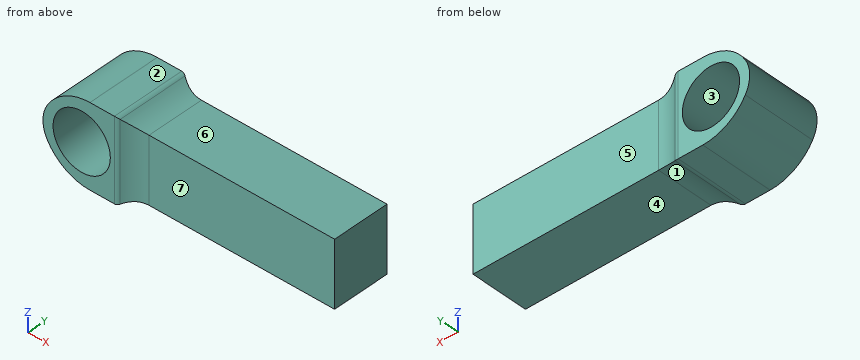
```python
from build123d import *

# Parameters (mm, degrees)
F0_W        = 10
F0_H        = 9
F1_DEPTH    = 5
F3_D        = 7
F4_T1_DEPTH = 39
F5_R        = 1
F6_W        = 7
F6_H        = 8
F7_DEPTH    = 25
F8_R        = 5
F9_R        = 4


# Not quite as in the source:
# - a fillet or chamfer that OpenCascade refuses, or shapes differently, is made with other operations: its cross-section is extruded or revolved along the edge and cut away or added


with BuildPart() as f1:
    # F0 (on Top) → F1 (new body, symmetric)
    with BuildSketch(Plane.XY):
        Rectangle(F0_W, F0_H)
    extrude(amount=F1_DEPTH, both=True)

    # F3 (through all)
    with Locations(Plane(origin=(0, 4.5, 0), x_dir=(-1, 0, 0), z_dir=(0, 1, 0))):
        with Locations((0, 0)):
            Hole(F3_D / 2)

    # F4: fillet of radius 6 on 2 edges, made by hand

    # F4_s2 → F4_t1 (cut)
    with BuildSketch(Plane.XZ.offset(-19.5)):
        with BuildLine():
            ThreePointArc((-5, -1), (-3.2426406871, 3.2426406871), (1, 5))
            Line((1, 5), (-5, 5))
            Line((-5, 5), (-5, -1))
        make_face()
        with BuildLine():
            ThreePointArc((1, -5), (-3.2426406871, -3.2426406871), (-5, 1))
            Line((-5, 1), (-5, -5))
            Line((-5, -5), (1, -5))
        make_face()
    extrude(amount=F4_T1_DEPTH, mode=Mode.SUBTRACT)

    # F5
    f5_edges = [f1.edges().sort_by_distance(p)[0] for p in [
        (5, -4.5, 0),
        (5, 0, -5),
        (5, 4.5, 0),
        (5, 0, 5),
    ]]
    fillet(f5_edges, radius=F5_R)

    # F6 (on face) → F7 (join)
    with BuildSketch(Plane.YZ.offset(5)):
        Rectangle(F6_W, F6_H)
    extrude(amount=F7_DEPTH)

    # F8
    f8_edges = [f1.edges().sort_by_distance(p)[0] for p in [
        (5, 0, 4),
        (5, -3.5, 0),
        (5, 3.5, 0),
        (5, 0, -4),
    ]]
    fillet(f8_edges, radius=F8_R)

    # F9
    f9_edges = [f1.edges().sort_by_distance(p)[0] for p in [
        (-4.91608, 0, 0),
    ]]
    fillet(f9_edges, radius=F9_R)


solid = f1.part
```
Geometry: final body of the model. Coordinates: model frame, mm. Face numbers are marked on the shaded views. A direction names the side the tool comes from. Coordinates: 2 decimals unless noted, no trailing zeros. Order: outer loops, then holes, each group sorted by start corner. A loop starts at its lowest first (then second) coordinate and runs counter-clockwise, first axis right, second up. Notation, with made-up numbers: (18.25, 46) - (36.25, 46) arc R14 cw to (36.25, 50) - close; hole circle Ø10 at (27, -13.5). An arc over 180 degrees is marked (long way). Write each question's results on one line, items separated by ' | '.
1) Line query: line 1 (Y direction, x = 26, z = -1.5); line 2 (Z direction, x = 25.5, y = -3); line 3 (Z direction, x = 0, y = 1). Output: solid intervals per line, ascending. Write a range as from..to.
Results list:
line 1: -3.5..3.5 | line 2: -4..4 | line 3: -4.92..-3.5, 3.5..4.92
2) Section A-A, the plane x = 0. Return loops of the section in (y, z).
Results list:
outline: (-4.5, -4.92) - (4.5, -4.92) - (4.5, -3.5) - (-4.5, -3.5) - close; (-4.5, 3.5) - (4.5, 3.5) - (4.5, 4.92) - (-4.5, 4.92) - close
3) Pull-direction query (Z, two-part tool) for the marked faces 1, 2 and 3; classes: pulls with the +Z half, pulls with the -Z half, needs draft (parallel to the pull), parting line crosses it, or undercut.
Results list:
face 1: pulls with the -Z half | face 2: pulls with the +Z half | face 3: undercut
4) Section B-B, the plane x = 25.5. Return loops of the section in (y, z), plus the area to 3 significant figures.
Results list:
outline: (-3.5, -4) - (3.5, -4) - (3.5, 4) - (-3.5, 4) - close | area: 56.0 mm^2
5) Pin query (flat end, axial travel): pin 1 (2.5 mm diameter, centred on x = 15.5, z = -1, fed in from +Y); pin 2 (2 mm diameter, centred on x = 23.5, y = -1, fed in from +Z); pin 3 (3.5 mm diameter, centred on x = 19.5, y = -0.5, fed in from -Z); pin 4 (4 mm diameter, centred on x = 6, y = 0, fed in from -Z). Return the tip coordinate at first contact, or that it passes through.
Results list:
pin 1: y = 3.5 | pin 2: z = 4 | pin 3: z = -4 | pin 4: z = -5
6) Set-up query: the marked faces 4, 5, 6 and 7. Return all of +Z, -Z, +X, -X, +Y, -Y with unobstructed straight access to the full face (end or side cutting, diameter ignored); none if empty.
Results list:
face 4: -Z, +X, +Y, -Y | face 5: +Z, -Z, +X, +Y | face 6: +Z, +X, +Y, -Y | face 7: +Z, -Z, +X, -Y
